from build123d import *

# Parameters (mm, degrees)
F0_W      = 170
F0_H      = 76
F1_DEPTH  = 30
F2_W      = 164
F2_H      = 70
F3_DEPTH  = 27
F6_W      = 166
F6_H      = 72
F6_W_2    = 164
F6_H_2    = 70
F7_DEPTH  = 2
F5_R      = 4
F9_DEPTH  = 3
F8_R      = 3.5
F10_DEPTH = 10
F11_R     = 0.5
F12_DEPTH = 0.5
F13_W     = 13
F13_H     = 5.5
F14_DEPTH = 3
F15_R     = 5
F16_W     = 19
F16_H     = 26
F17_DEPTH = 25
F18_W     = 32
F18_H     = 40
F18_W_2   = 19
F18_H_2   = 26
F19_DEPTH = 1


with BuildPart() as f1:
    # F0 (on Top) → F1 (new body)
    with BuildSketch(Plane.XY):
        with Locations((85, 38)):
            Rectangle(F0_W, F0_H)
    extrude(amount=F1_DEPTH)

    # F2 (on face) → F3 (cut)
    with BuildSketch(Plane.XY.offset(30)):
        with Locations((85, 38)):
            Rectangle(F2_W, F2_H)
    extrude(amount=-F3_DEPTH, mode=Mode.SUBTRACT)

    # F6 (on face) → F7 (join)
    with BuildSketch(Plane.XY.offset(30)):
        with Locations((85, 38)):
            Rectangle(F6_W, F6_H)
        with Locations((85, 38)):
            Rectangle(F6_W_2, F6_H_2, mode=Mode.SUBTRACT)
    extrude(amount=F7_DEPTH)

    # F5 (on face) → F9 (cut, through all)
    with BuildSketch(Plane(origin=(0, 0, 0), x_dir=(0, -1, 0), z_dir=(-1, 0, 0))):
        with Locations((-57, 18)):
            Circle(F5_R)
        with Locations((-19, 18)):
            Circle(F5_R)
    extrude(amount=-F9_DEPTH, mode=Mode.SUBTRACT)

    # F8 (on face) → F10 (join)
    with BuildSketch(Plane.XY.offset(3)):
        with Locations((8, 68)):
            Circle(F8_R)
        with Locations((8, 8)):
            Circle(F8_R)
        with Locations((162, 8)):
            Circle(F8_R)
        with Locations((162, 68)):
            Circle(F8_R)
    extrude(amount=F10_DEPTH)

    # F11 (on face) → F12 (cut)
    with BuildSketch(Plane.XY.offset(13)):
        with Locations((162, 8)):
            Circle(F11_R)
        with Locations((8, 8)):
            Circle(F11_R)
        with Locations((8, 68)):
            Circle(F11_R)
        with Locations((162, 68)):
            Circle(F11_R)
    extrude(amount=-F12_DEPTH, mode=Mode.SUBTRACT)

    # F13 (on face) → F14 (cut, through all)
    with BuildSketch(Plane.YZ.offset(170)):
        with Locations((38, 18)):
            Rectangle(F13_W, F13_H)
    extrude(amount=-F14_DEPTH, mode=Mode.SUBTRACT)

    # F15
    f15_edges = [f1.edges().sort_by_distance(p)[0] for p in [
        (0, 38, 0),
        (85, 76, 0),
        (170, 38, 0),
        (85, 0, 0),
        (170, 76, 15),
        (170, 0, 15),
        (0, 76, 15),
        (0, 0, 15),
    ]]
    fillet(f15_edges, radius=F15_R)

    # F16 (on face) → F17 (cut)
    with BuildSketch(Plane.XY.offset(3)):
        with Locations((22.5, 38)):
            Rectangle(F16_W, F16_H)
    extrude(amount=-F17_DEPTH, mode=Mode.SUBTRACT)

    # F18 (on face) → F19 (cut)
    with BuildSketch(Plane.XY.offset(3)):
        with Locations((24, 38)):
            Rectangle(F18_W, F18_H)
        with Locations((22.5, 38)):
            Rectangle(F18_W_2, F18_H_2, mode=Mode.SUBTRACT)
    extrude(amount=-F19_DEPTH, mode=Mode.SUBTRACT)


solid = f1.part
Could you check a few things on this model? Use its own coordinates, in mm. A direction names the side the tool comes from. Coordinates: 2 decimals unless noted, no trailing zeros. Loops run counter-clockwise (first coordinate to the right, second up) from the corner with the lowest first, then second, coordinate; pieces in that order, holes last.
1. For faces 5 (the face through (84, 0, 17)), 6 (the face through (162, 67, 13)), 7 (the face through (169, 38, 15.25)), which set-ups out of +Z, -Z, +X, -X, +Y, -Y let a thin tool reach every point of the face, with its end or its side?
2. Imagine slicing it at C-C (z = 18). Please give me the cut outline in (x, y).
3. Imagine slicing it at A-A (y = 39.5). Please give me the cut outline in (x, z), and give its area (3 significant figures).
4. We'd pull the mould along X, two halves only. Please class faces 1 (the face through (169, 38, 2)), 2 (the face through (169, 31.5, 18)), 3 (the face through (1, 2, 18)), 4 (the face through (34, 38, 2)): released by +X, released by -X, zero draft, split by the parting line, or undercut.
5. For P1, Ø3, axis at x = 105.5, y = 55.5, coming from the +Z side; P2, Ø0.6, axis at x = 22, z = 1, coming from the -Y side; P3, Ø2, axis at y = 30, z = 3.5, coming from the +X side, each with a flat end and sliding along its axis, tell me the tip position at first contact or that it passes through.
6. Imagine slicing it at B-B (z = 26). Please give me the cut outline in (x, y), and give its area (3 significant figures).
7. Imagine slicing it at D-D (x = 25.5). Please give me the cut outline in (y, z), and give its area (3 significant figures).
8. I need wall thicknesses on L1, parallel to Y at x = 8, z = 12.75; L2, parallel to X at y = 5, z = 14.5; L3, parallel to X at y = 29.5, z = 30.5. Which ranges of each line are inside material? Lowest first, please.
Computed values:
1. face 5: +Z, -Z, +X, -X, -Y
1. face 6: +Z
1. face 7: +X
2. outline: (0, 5) arc R5 ccw to (5, 0) - (165, 0) arc R5 ccw to (170, 5) - (170, 31.5) - (167, 31.5) - (167, 3) - (3, 3) - (3, 15) - (0, 15) - close; (0, 23) - (3, 23) - (3, 53) - (0, 53) - close; (0, 61) - (3, 61) - (3, 73) - (167, 73) - (167, 44.5) - (170, 44.5) - (170, 71) arc R5 ccw to (165, 76) - (5, 76) arc R5 ccw to (0, 71) - close
3. outline: (0, 5) arc R5 ccw to (5, 0) - (13, 0) - (13, 2) - (8, 2) - (8, 3) - (3, 3) - (3, 32) - (2, 32) - (2, 30) - (0, 30) - close; (32, 0) - (165, 0) arc R5 ccw to (170, 5) - (170, 15.25) - (167, 15.25) - (167, 3) - (40, 3) - (40, 2) - (32, 2) - close; (167, 20.75) - (170, 20.75) - (170, 30) - (168, 30) - (168, 32) - (167, 32) - close
3. area: 579 mm2
4. face 1: released by +X
4. face 2: zero draft
4. face 3: released by -X
4. face 4: undercut
5. P1: stops at z = 3
5. P2: stops at y = 1.64
5. P3: stops at x = 169.97
6. outline: (0, 5) arc R5 ccw to (5, 0) - (165, 0) arc R5 ccw to (170, 5) - (170, 71) arc R5 ccw to (165, 76) - (5, 76) arc R5 ccw to (0, 71) - close; hole (3, 3) - (167, 3) - (167, 73) - (3, 73) - close
6. area: 1,420 mm2
7. outline: (0, 5) arc R5 ccw to (5, 0) - (25, 0) - (25, 2) - (18, 2) - (18, 3) - (3, 3) - (3, 32) - (2, 32) - (2, 30) - (0, 30) - close; (51, 0) - (71, 0) arc R5 ccw to (76, 5) - (76, 30) - (74, 30) - (74, 32) - (73, 32) - (73, 3) - (58, 3) - (58, 2) - (51, 2) - close
7. area: 291 mm2
8. L1: y = 0 to 3, 4.5 to 7.5, 8.5 to 11.5, 64.5 to 67.5, 68.5 to 71.5, 73 to 76
8. L2: x = 0 to 3, 167 to 170
8. L3: x = 2 to 3, 167 to 168
